Geometry check sheet. Reference: the model listing, model coordinates, mm. Give positions to 0.01 mm unless a question says otherwise; leave off trailing zeros. Write each loop counter-clockwise with the first axis right and the second up, starting at its lowest first coordinate (ties: lowest second). Pieces come first, ordered by that corner, then holes. Notation, with made-up numbers: M 58.5,17.5 L 99.5,17.5 A20 ccw 99.5,48.5 Z; hole C -26.75,-20 d10. An arc over 180 degrees is marked long. Write each question's results on one line, items separated by ' | '.
```python
from build123d import *

# Parameters (mm, degrees)
SKETCH1_W           = 40
SKETCH1_H           = 100
SKETCH1_H_2         = 60
BOSS_EXTRUDE1_DEPTH = 2
SKETCH2_R           = 3
CUT_EXTRUDE1_DEPTH  = 79.204859184
CHAMFER1_SIZE       = 3


# Read off the part's stored shape, not the designer's step: Mirror2
with BuildPart() as part:
    # Sketch1 → Boss-Extrude1 (new, symmetric)
    with BuildSketch(Plane.XY):
        Rectangle(SKETCH1_W, SKETCH1_H)
        with Locations((40, 0)):
            Rectangle(SKETCH1_W, SKETCH1_H_2)
        Polygon((60, 30), (20, 50), (20, 30), align=None)
        Polygon((20, -30), (20, -50), (60, -30), align=None)
    extrude(amount=BOSS_EXTRUDE1_DEPTH, both=True)

    # Sketch2 → Cut-Extrude1 (cut, through all)
    with BuildSketch(Plane.XY.offset(2)):
        with Locations((50, 20)):
            Circle(SKETCH2_R)
        with Locations((30, 20)):
            Circle(SKETCH2_R)
        with Locations((-10, 0)):
            Circle(SKETCH2_R)
        with Locations((10, 0)):
            Circle(SKETCH2_R)
        with Locations((-10, 40)):
            Circle(SKETCH2_R)
        with Locations((10, 40)):
            Circle(SKETCH2_R)
    extrude(amount=-CUT_EXTRUDE1_DEPTH, mode=Mode.SUBTRACT)

    # Chamfer1
    chamfer1_edges = [part.edges().sort_by_distance(p)[0] for p in [
        (47, 20, 2),
        (7, 40, 2),
        (27, 20, 2),
        (-13, 0, 2),
        (7, 0, 2),
        (-13, 40, 2),
    ]]
    chamfer(chamfer1_edges, length=CHAMFER1_SIZE)

    # Mirror2 outline → Mirror2 (revolve, cut)
    with BuildSketch(Plane(origin=(-10, -40, 0), x_dir=(1, 0, 0), z_dir=(0, -1, 0))):
        Polygon((0, -2), (3, -2), (3, -1), (6, 2), (0, 2), align=None)
    revolve(axis=Axis((-10, -40, 0), (0, 0, 1)), mode=Mode.SUBTRACT)

    # Mirror2 2 outline → Mirror2 2 (revolve, cut)
    with BuildSketch(Plane(origin=(50, -20, 0), x_dir=(1, 0, 0), z_dir=(0, -1, 0))):
        Polygon((0, -2), (3, -2), (3, -1), (6, 2), (0, 2), align=None)
    revolve(axis=Axis((50, -20, 0), (0, 0, 1)), mode=Mode.SUBTRACT)

    # Mirror2 3 outline → Mirror2 3 (revolve, cut)
    with BuildSketch(Plane(origin=(30, -20, 0), x_dir=(1, 0, 0), z_dir=(0, -1, 0))):
        Polygon((0, -2), (3, -2), (3, -1), (6, 2), (0, 2), align=None)
    revolve(axis=Axis((30, -20, 0), (0, 0, 1)), mode=Mode.SUBTRACT)

    # Mirror2 4 outline → Mirror2 4 (revolve, cut)
    with BuildSketch(Plane(origin=(10, -40, 0), x_dir=(1, 0, 0), z_dir=(0, -1, 0))):
        Polygon((0, -2), (3, -2), (3, -1), (6, 2), (0, 2), align=None)
    revolve(axis=Axis((10, -40, 0), (0, 0, 1)), mode=Mode.SUBTRACT)


solid = part.part
```
Q1. Release check for a two-part mould opening along Y. For faces 1 (the face through (27.47, -21.94, -0.81)), 2 (the face through (0, 50, 0)), 3 (the face through (0, -50, 0)) record: released by +Y, released by -Y, zero draft, split by the parting line, or undercut.
Answer key:
face 1: undercut | face 2: released by +Y | face 3: released by -Y
Q2. Section check B-B (x = -10). Enter the section's corners in (y, z).
Answer key:
outline: M -50,-2 L -43,-2 L -43,-1 L -46,2 L -50,2 Z; M -37,-2 L -3,-2 L -3,-1 L -6,2 L -34,2 L -37,-1 Z; M 3,-2 L 37,-2 L 37,-1 L 34,2 L 6,2 L 3,-1 Z; M 43,-2 L 50,-2 L 50,2 L 46,2 L 43,-1 Z
Q3. Depth check by flat-ended pin: P1, Ø5.5, axis at x = 50, y = -20, coming from the +Z side; P2, Ø7, axis at x = -10, y = 40, coming from the +Z side; P3, Ø9.5, axis at x = 50, y = 20, coming from the -Z side; P4, Ø8, axis at x = 10, y = 40, coming from the +Z side. Enter the tip coordinate at first touch or a pass-through.
Answer key:
P1: passes through | P2: stops at z = -0.5 | P3: stops at z = -2 | P4: stops at z = 0
Q4. Section check C-C (z = -0.25). State how many separate pieces and enclosed holes the cut face has, then the cut area to 3 significant figures.
Answer key:
separate pieces: 1 | enclosed holes: 10 | area: 6,760 mm2
Q5. Section check A-A (y = -40). Enter the section's corners in (x, z).
Answer key:
outline: M -20,-2 L -13,-2 L -13,-1 L -16,2 L -20,2 Z; M -7,-2 L 7,-2 L 7,-1 L 4,2 L -4,2 L -7,-1 Z; M 13,-2 L 40,-2 L 40,2 L 16,2 L 13,-1 Z
Q6. Section check D-D (x = 50). Enter the section's corners in (y, z), then the cut area to 3 significant figures.
Answer key:
outline: M -35,-2 L -23,-2 L -23,-1 L -26,2 L -35,2 Z; M -17,-2 L 17,-2 L 17,-1 L 14,2 L -14,2 L -17,-1 Z; M 23,-2 L 35,-2 L 35,2 L 26,2 L 23,-1 Z | area: 214 mm2
Q7. Material ranges on probe 1 along Y at (x, z) = (-10, -1.3); probe 2 along Y at (x, z) = (50, -1.3); probe 3 along Y at (x, z) = (-9, 1.85), recorded low to high. Write a range as [from, to].
Answer key:
probe 1: y = [-50, -43], [-37, -3], [3, 37], [43, 50] | probe 2: y = [-35, -23], [-17, 17], [23, 35] | probe 3: y = [-50, -45.76], [-34.24, -5.76], [5.76, 34.24], [45.76, 50]
